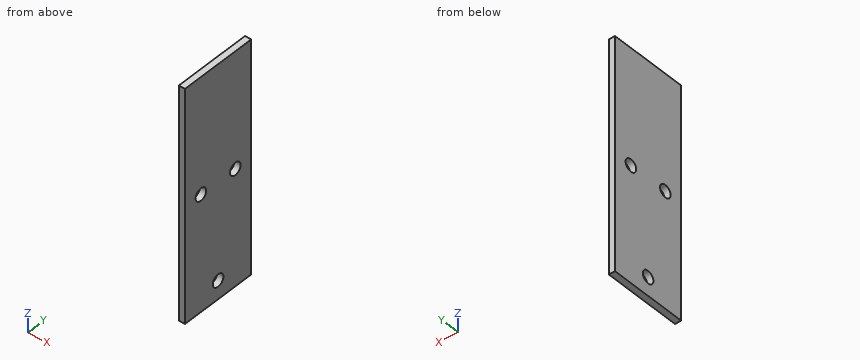
from build123d import *

# Parameters (mm, degrees)
SKETCH1_W           = 4
SKETCH1_H           = 150
BOSS_EXTRUDE1_DEPTH = 50
SKETCH2_R           = 4
CUT_EXTRUDE1_DEPTH  = 10


with BuildPart() as part:
    # Sketch1 → Boss-Extrude1 (new body)
    with BuildSketch(Plane(origin=(0, 0, 0), x_dir=(1, 0, 0), z_dir=(0, 1, 0))):
        Rectangle(SKETCH1_W, SKETCH1_H)
    extrude(amount=BOSS_EXTRUDE1_DEPTH)

    # Sketch2 → Cut-Extrude1 (cut)
    with BuildSketch(Plane.ZY.offset(2)):
        with Locations((0, 38)):
            Circle(SKETCH2_R)
        with Locations((0, 12)):
            Circle(SKETCH2_R)
        with Locations((-63, 25)):
            Circle(SKETCH2_R)
    extrude(amount=-CUT_EXTRUDE1_DEPTH, mode=Mode.SUBTRACT)


solid = part.part
Geometry: final body of the model. Coordinates: model frame, mm. Round coordinates to 2 decimals unless told otherwise and drop trailing zeros. Loops run counter-clockwise (first coordinate to the right, second up) from the corner with the lowest first, then second, coordinate; pieces in that order, holes last.
Q1. Section C-C on z = -63. Return loops of the section in (x, y).
Q2. Material intervals for L1, parallel to Y at x = -0.8, z = 0; L2, parallel to Y at x = -0.25, z = -1; L3, parallel to Z at x = 0.15, y = 36, sorted ascending.
Q3. Section B-B on z = 0. Return loops of the section in (x, y).
Q4. Pin query (flat end, axial travel): P1, Ø13, axis at y = 12, z = 0, coming from the -X side. Return the tip coordinate at first contact, or that it passes through.
Q5. Section A-A on y = 12. Return loops of the section in (x, z).
Q6. Section D-D on x = -0.5. Return loops of the section in (y, z).
Evaluation:
1. outline: (-2, 0) - (2, 0) - (2, 21) - (-2, 21) - close; (-2, 29) - (2, 29) - (2, 50) - (-2, 50) - close
2. L1: y = 0 to 8, 16 to 34, 42 to 50
2. L2: y = 0 to 8.13, 15.87 to 34.13, 41.87 to 50
2. L3: z = -75 to -3.46, 3.46 to 75
3. outline: (-2, 0) - (2, 0) - (2, 8) - (-2, 8) - close; (-2, 16) - (2, 16) - (2, 34) - (-2, 34) - close; (-2, 42) - (2, 42) - (2, 50) - (-2, 50) - close
4. P1: stops at x = -2
5. outline: (-2, -75) - (2, -75) - (2, -4) - (-2, -4) - close; (-2, 4) - (2, 4) - (2, 75) - (-2, 75) - close
6. outline: (0, -75) - (50, -75) - (50, 75) - (0, 75) - close; hole circle Ø8 at (12, 0); hole circle Ø8 at (25, -63); hole circle Ø8 at (38, 0)
